Design review of the part built by this model. Coordinates are the model's own, in mm. Face numbers are marked on the shaded views. A direction names the side the tool comes from. Coordinates: 2 decimals unless noted, no trailing zeros. Write each loop counter-clockwise with the first axis right and the second up, starting at its lowest first coordinate (ties: lowest second). Pieces come first, ordered by that corner, then holes. Notation, with made-up numbers: (89.25, 65) - (102.25, 65) arc R34 cw to (102.25, 100) - close; hole circle Ø9 at (-25.5, -14). An arc over 180 degrees is marked (long way). Use a Markdown table: item, result.
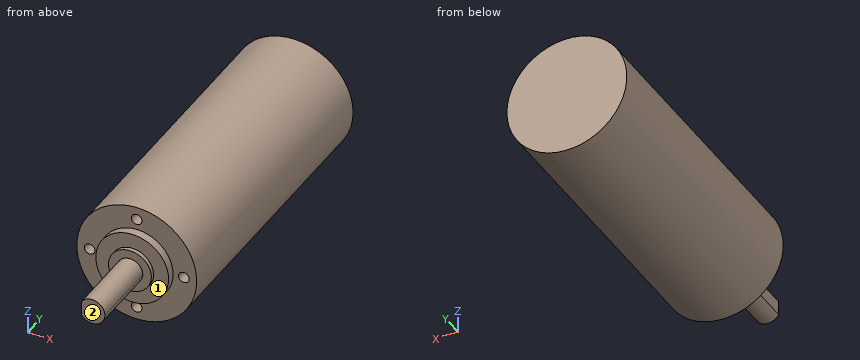
from build123d import *

# Parameters (mm, degrees)
F0_R     = 13.9954
F1_DEPTH = 31.496
F2_DEPTH = 37.4904
F4_DEPTH = 19.7104
F3_R     = 5.0038
F5_DEPTH = 2.9972
F3_R_2   = 8.4963
F6_DEPTH = 2.0066
F7_D     = 2.4892
F7_DEPTH = 5.9944
F7_TIP   = 0.7478311264


with BuildPart() as f1:
    # F0 (on Front) → F1 (new body)
    with BuildSketch(Plane.XZ):
        Circle(F0_R)
    extrude(amount=F1_DEPTH)

    # F2 (add): a face of the model
    f2_faces = [f1.faces().sort_by_distance(p)[0] for p in [
        (0, 0, 0),
    ]]
    extrude(f2_faces, amount=F2_DEPTH)

    # F3 (on face) → F4 (join)
    with BuildSketch(Plane.XZ.offset(31.496)):
        with BuildLine():
            ThreePointArc((-2.5146, -1.6309490121), (0.8504259874, -2.8740186986), (2.9972, 0))
            ThreePointArc((2.9972, 0), (0.8504259874, 2.8740186986), (-2.5146, 1.6309490121))
            Line((-2.5146, 1.6309490121), (-2.5146, -1.6309490121))
        make_face()
    extrude(amount=F4_DEPTH)

    # F3 (on face) → F5 (join)
    with BuildSketch(Plane.XZ.offset(31.496)):
        Circle(F3_R)
        with BuildLine():
            ThreePointArc((-2.5146, 1.6309490121), (0.8504259874, 2.8740186986), (2.9972, 0))
            ThreePointArc((2.9972, 0), (0.8504259874, -2.8740186986), (-2.5146, -1.6309490121))
            ThreePointArc((-2.5146, -1.6309490121), (-2.9972, 0), (-2.5146, 1.6309490121))
        make_face(mode=Mode.SUBTRACT)
        with BuildLine():
            Line((-2.5146, -1.6309490121), (-2.5146, 1.6309490121))
            ThreePointArc((-2.5146, 1.6309490121), (-2.9972, 0), (-2.5146, -1.6309490121))
        make_face()
    extrude(amount=F5_DEPTH)

    # F3 (on face) → F6 (join)
    with BuildSketch(Plane.XZ.offset(31.496)):
        Circle(F3_R_2)
        Circle(F3_R, mode=Mode.SUBTRACT)
    extrude(amount=F6_DEPTH)

    # F7
    with Locations(Plane.XZ.offset(31.496)):
        with Locations((10.9982, 0), (0, -10.9982), (0, 10.9982), (-10.9982, 0)):
            Hole(F7_D / 2, depth=F7_DEPTH)
            with Locations((0, 0, -(F7_DEPTH + F7_TIP / 2))):  # 118° drill point
                Cone(0, F7_D / 2, F7_TIP, mode=Mode.SUBTRACT)


solid = f1.part
(1) Take a section at A-A on z = -6.25. Write out the cut boundary in (x, y).
Determined:
| item | result |
|---|---|
| outline | (-12.52, -31.5) - (-5.76, -31.5) - (-5.76, -33.5) - (5.76, -33.5) - (5.76, -31.5) - (12.52, -31.5) - (12.52, 37.49) - (-12.52, 37.49) - close |
(2) For pin 1 (6 mm diameter, centred on y = -27, z = -10.5, fed in from -X); pin 2 (3.5 mm diameter, centred on y = -43, z = 0.5, fed in from -X); pin 3 (2 mm diameter, centred on x = 0, z = 11, fed in from -Y); pin 4 (11 mm diameter, centred on x = 2, z = -2.5, fed in from -Y), all flat-tipped, find the tip position at first contact; note any pin that passes through.
Determined:
| item | result |
|---|---|
| pin 1 | x = -11.82 |
| pin 2 | x = -2.51 |
| pin 3 | y = -25.36 |
| pin 4 | y = -51.21 |
(3) Machinability: for the marked faces 1 and 2, which of the approach directions +Z, -Z, +X, -X, +Y, -Y give a long, thin tool a straight path to every point of the face, cutting with its end or side? Answer none if there is none.
Determined:
| item | result |
|---|---|
| face 1 | -Y |
| face 2 | +Z, -Z, +X, -X, -Y |
(4) For L1, parallel to Z at x = 0, y = -29.95; L2, parallel to Y at x = -5.5, z = 7; L3, parallel to Y at x = 8.25, z = -1.75, list the stretches that pass through material, from the lowest coordinate up. Write a range as from..to.
Determined:
| item | result |
|---|---|
| L1 | -14..-12.24, -9.75..9.75, 12.24..14 |
| L2 | -31.5..37.49 |
| L3 | -33.5..37.49 |
(5) Take a section at B-B on y = 32.5. Write out the cut boundary in (x, z), and give its area (3 significant figures).
Determined:
| item | result |
|---|---|
| outline | circle Ø27.99 at (0, 0) |
| area | 615 mm2 |
